Autodesk Inventor part; units mm, degrees
ref_plane "YZ Plane" through (0, 0, 0) normal (1, 0, 0) x (0, 1, 0)
ref_plane "XZ Plane" through (0, 0, 0) normal (0, 1, 0) x (-1, 0, 0)
ref_plane "XY Plane" through (0, 0, 0) normal (0, 0, 1) x (1, 0, 0)
sketch "Sketch1" plane through (0, 0, 0) normal (1, 0, 0) x (0, 1, 0)
  line L0 (0.3153, 51.2567) -> (-2.5847, 51.2567)
  line L1 (-2.5847, 51.2567) -> (-2.5847, -10.8433)
  line L2 (-2.5847, -10.8433) -> (0.3153, -10.8433)
  line L3 (0.3153, -10.8433) -> (0.3153, 51.2567)
  arc A0 (0.3153, 51.2567) -> (-0.0756, 57.3616) centre (-1.1163, 54.23) ccw
  arc A1 (-2.2756, 57.3196) -> (-2.5847, 51.2567) centre (-1.1371, 54.2222) ccw
  line L4 (-2.2756, 57.3196) -> (-2.2756, 56.2196)
  line L5 (-0.0756, 57.3616) -> (-0.0756, 56.2616)
  arc A2 (-2.2756, 56.2196) -> (-0.0756, 56.2616) centre (-1.1371, 54.2222) ccw
  arc A3 (-2.5847, -10.8433) -> (-2.5847, -16.9063) centre (-1.2354, -13.8748) ccw
  arc A4 (-0.3847, -16.0719) -> (-2.5847, -15.8063) centre (-1.2354, -13.8748) ccw
  arc A5 (-0.3847, -17.1719) -> (0.3153, -10.8433) centre (-1.2354, -13.8748) ccw
  line L6 (-2.5847, -15.8063) -> (-2.5847, -16.9063)
  line L7 (-0.3847, -16.0719) -> (-0.3847, -17.1719)
  point P0 (0, 0)
  dimension "d0" = 2.9
  dimension "d1" = 62.1
  dimension "d163" = 1.1
  dimension "d164" = 1.1
  dimension "d165" = 2.2
  dimension "d166" = 2.2991
  dimension "d167" = 3.3
  dimension "d168" = 3.3
  dimension "d171" = 6.063
  dimension "d172" = 6.1049
  dimension "d174" = 6.063
  dimension "d176" = 1.1
  dimension "d177" = 1.1
  dimension "d178" = 2.2
extrude "Extrusion1" add sketch "Sketch1" against normal blind 20
sketch "Sketch3" plane through (0, 0, 0) normal (1, 0, 0) x (0, 0, -1)
  line L0 (10.8433, -2.5847) -> (-51.2567, -2.5847)
  line L1 (-51.2567, 0.3153) -> (10.8433, 0.3153)
  line L2 (10.8433, 0.3153) -> (10.8433, -2.5847)
  line L3 (10.8433, -2.5847) -> (-51.2567, -2.5847)
  line L4 (-51.2567, -2.5847) -> (-51.2567, 0.3153)
  point P0 (0, 0)
extrude "Extrusion2" add sketch "Sketch3" along normal blind 42.1
sketch "Sketch4" plane through (42.1, 0, 0) normal (1, 0, 0) x (0, 0, -1)
  line L0 (10.8433, -2.5847) -> (-51.2567, -2.5847)
  line L1 (10.8433, -2.5847) -> (-51.2567, -2.5847)
  line L2 (-51.2567, -2.5847) -> (-51.2567, 0.3153)
  line L3 (-51.2567, 0.3153) -> (10.8433, 0.3153)
  line L4 (10.8433, 0.3153) -> (10.8433, -2.5847)
  arc A0 (-57.3196, -2.2756) -> (-51.2567, -2.5847) centre (-54.2222, -1.1371) ccw
  arc A1 (-57.3196, -2.2756) -> (-51.2567, -2.5847) centre (-54.2222, -1.1371) ccw
  arc A2 (-51.2567, 0.3153) -> (-57.3616, -0.0756) centre (-54.23, -1.1163) ccw
  arc A3 (-51.2567, 0.3153) -> (-57.3616, -0.0756) centre (-54.2286, -1.1372) ccw
  arc A4 (-56.2196, -2.2756) -> (-56.2616, -0.0756) centre (-54.2222, -1.1371) ccw
  arc A5 (-56.2196, -2.2756) -> (-56.2616, -0.0756) centre (-54.2286, -1.1372) ccw
  line L5 (-56.2196, -2.2756) -> (-57.3196, -2.2756)
  line L6 (-56.2196, -2.2756) -> (-57.3196, -2.2756)
  line L7 (-57.3616, -0.0756) -> (-56.2616, -0.0756)
  line L8 (-56.2616, -0.0756) -> (-57.3616, -0.0756)
  arc A6 (-57.3196, -2.2756) -> (-51.2567, -2.5847) centre (-54.2222, -1.1371) ccw
  line L9 (-51.2567, -2.5847) -> (-51.2567, 0.3153)
  arc A7 (-51.2567, 0.3153) -> (-57.3616, -0.0756) centre (-54.23, -1.1163) ccw
  arc A8 (-56.2196, -2.2756) -> (-56.2616, -0.0756) centre (-54.2222, -1.1371) ccw
  line L10 (-57.3196, -2.2756) -> (-56.2196, -2.2756)
  line L11 (-56.2616, -0.0756) -> (-57.3616, -0.0756)
  line L12 (-56.2616, -0.0756) -> (-57.3616, -0.0756)
  line L13 (-56.2616, -0.0756) -> (-57.3616, -0.0756)
  arc A9 (10.8433, -2.5847) -> (16.9063, -2.5847) centre (13.8748, -1.2354) ccw
  arc A10 (10.8433, -2.5847) -> (16.9063, -2.5847) centre (13.8748, -1.2354) ccw
  arc A11 (17.1719, -0.3847) -> (10.8433, 0.3153) centre (13.8748, -1.2354) ccw
  arc A12 (17.1719, -0.3847) -> (10.8433, 0.3153) centre (13.8748, -1.2354) ccw
  arc A13 (16.0719, -0.3847) -> (15.8063, -2.5847) centre (13.8748, -1.2354) ccw
  arc A14 (16.0719, -0.3847) -> (15.8063, -2.5847) centre (13.8748, -1.2354) ccw
  line L14 (15.8063, -2.5847) -> (16.9063, -2.5847)
  line L15 (16.0719, -0.3847) -> (17.1719, -0.3847)
extrude "Extrusion3" add sketch "Sketch4" along normal blind 20 contours L0 L2 L3 L4 | L4 A11 L15 A13 L14 A9 | A0 L5 A4 L7 A3 L2 | A3 A2
sketch "Sketch9" plane through (0, -2.5847, 51.2567) normal (0, 0, 1) x (1, 0, 0)
  line L0 (0, 2.9) -> (42.1, 2.9)
  line L1 (0, 2.9) -> (42.1, 2.9)
  line L2 (42.1, 2.9) -> (42.1, 0)
  line L3 (42.1, 0) -> (0, 0)
  line L4 (0, 0) -> (0, 2.9)
  point P0 (0, 2.5847)
extrude "Extrusion4" add sketch "Sketch9" along normal blind 0.001
sketch "Sketch10" plane through (-20, 0, 0) normal (-1, 0, 0) x (0, 0, 1)
  arc A0 (51.2567, -2.5847) -> (57.3196, -2.2756) centre (54.2222, -1.1371) ccw
  line L0 (-10.8433, 0.3153) -> (-10.8433, -2.5847)
  line L1 (51.2567, -2.5847) -> (-10.8433, -2.5847)
  line L2 (-10.8433, -2.5847) -> (-10.8433, 0.3153)
  line L3 (-10.8433, 0.3153) -> (51.2567, 0.3153)
  line L4 (51.2567, 0.3153) -> (51.2567, -2.5847)
  point P0 (0, 0)
  point P1 (-10.8433, -2.5847)
extrude "Extrusion5" add sketch "Sketch10" along normal blind 8.95
sketch "Sketch11" plane through (62.1, 0, 0) normal (1, 0, 0) x (0, 0, -1)
  line L0 (10.8433, -2.5847) -> (10.8433, 0.3153)
  arc A0 (-51.2567, 0.3153) -> (-57.3616, -0.0756) centre (-54.23, -1.1163) ccw
  line L1 (10.8433, -2.5847) -> (-51.2567, -2.5847)
  line L2 (-51.2567, -2.5847) -> (-51.2567, 0.3153)
  line L3 (-51.2567, 0.3153) -> (10.8433, 0.3153)
  line L4 (10.8433, 0.3153) -> (10.8433, -2.5847)
  point P0 (0, 0)
  point P1 (-57.2033, 0.3153)
  point P2 (10.8433, 0.3153)
extrude "Extrusion6" add sketch "Sketch11" along normal blind 8.95
sketch "Sketch12" plane through (0, -2.5847, 57.2567) normal (0, -1, 0) x (1, 0, 0)
  line L0 (-20, -6) -> (-30, -6)
  line L1 (-30, -68.1) -> (-30, -6)
  point P0 (-24.59, -14.57)
  dimension "d133" = 8.57
  dimension "d134" = 5.41
hole "Hole5" at (-24.59, -2.5847, 42.6867) direction (0, 1, 0) diameter 2.921 end through all
sketch "Sketch13" plane through (0, -2.5847, 57.2567) normal (0, -1, 0) x (1, 0, 0)
  line L0 (0, -6) -> (-20, -6)
  circle A0 centre (-24.59, -14.57) radius 1.4605
  point P0 (-11.33, -14.57)
  dimension "d135" = 8.57
  dimension "d136" = 13.26
hole "Hole6" at (-11.33, -2.5847, 42.6867) direction (0, 1, 0) diameter 2.921 end through all
sketch "Sketch14" plane through (0, -2.5847, 57.2567) normal (0, -1, 0) x (1, 0, 0)
  line L0 (-28.95, -68.1) -> (-28.95, -6)
  circle A0 centre (-24.59, -14.57) radius 1.4605
  point P0 (0, -57.2567)
  point P1 (-23.54, -59.5177)
  dimension "d137" = 5.41
  dimension "d138" = 44.96
hole "Hole7" at (-23.54, -2.5847, -2.2611) direction (0, 1, 0) diameter 2.921 end through all
sketch "Sketch15" plane through (0, -2.5847, 57.2567) normal (0, -1, 0) x (1, 0, 0)
  circle A0 centre (-11.33, -14.57) radius 1.4605
  circle A1 centre (-23.54, -59.5177) radius 1.4605
  point P0 (0, -57.2567)
  point P1 (-10.28, -59.53)
  dimension "d139" = 44.96
  dimension "d148" = 13.26
hole "Hole8" at (-10.28, -2.5847, -2.2733) direction (0, 1, 0) diameter 2.921 end through all
sketch "Sketch17" plane through (0, -2.5847, 57.2567) normal (0, -1, 0) x (1, 0, 0)
  line L0 (71.05, -6) -> (71.05, -68.1)
  line L1 (62.1, -6) -> (71.05, -6)
  point P0 (0, -57.2567)
  point P1 (65.64, -14.57)
  dimension "d142" = 5.41
  dimension "d147" = 8.57
hole "Hole10" at (65.64, -2.5847, 42.6867) direction (0, 1, 0) diameter 2.921 end through all
sketch "Sketch16" plane through (0, -2.5847, 57.2567) normal (0, -1, 0) x (1, 0, 0)
  circle A0 centre (65.64, -14.57) radius 1.4605
  line L0 (42.1, -6) -> (62.1, -6)
  point P0 (0, -57.2567)
  point P1 (52.38, -14.57)
  dimension "d144" = 13.26
  dimension "d146" = 8.57
hole "Hole9" at (52.38, -2.5847, 42.6867) direction (0, 1, 0) diameter 2.921 end through all
sketch "Sketch19" plane through (0, -2.5847, 57.2567) normal (0, -1, 0) x (1, 0, 0)
  circle A0 centre (65.64, -14.57) radius 1.4605
  line L0 (71.05, -6) -> (71.05, -68.1)
  point P0 (0, -57.2567)
  point P1 (65.64, -59.53)
  dimension "d141" = 44.96
  dimension "d143" = 5.41
hole "Hole12" at (65.64, -2.5847, -2.2733) direction (0, 1, 0) diameter 2.921 end through all
sketch "Sketch18" plane through (0, -2.5847, 57.2567) normal (0, -1, 0) x (1, 0, 0)
  circle A0 centre (52.38, -14.57) radius 1.4605
  circle A1 centre (65.64, -59.53) radius 1.4605
  point P0 (0, -57.2567)
  point P1 (52.38, -59.53)
  dimension "d140" = 44.96
  dimension "d145" = 13.26
hole "Hole11" at (52.38, -2.5847, -2.2733) direction (0, 1, 0) diameter 2.921 end through all
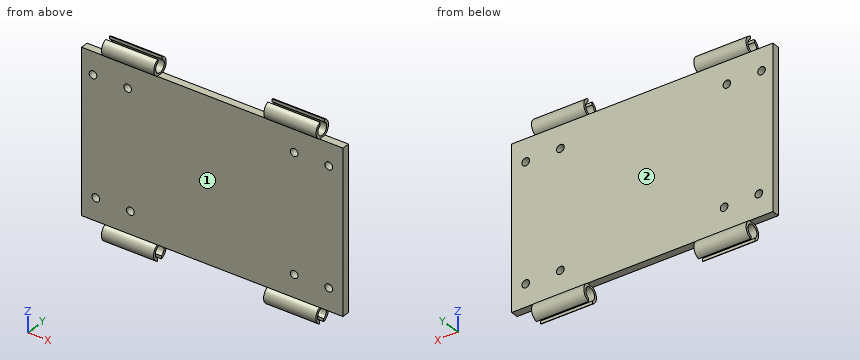
Design review of the part built by this model. Coordinates are the model's own, in mm. Face numbers are marked on the shaded views. A direction names the side the tool comes from. Coordinates: 2 decimals unless noted, no trailing zeros. Order: outer loops, then holes, each group sorted by start corner. A loop starts at its lowest first (then second) coordinate and runs counter-clockwise, first axis right, second up.
Item 1: For line 1 (Z direction, x = 65.64, y = -1.1); line 2 (Z direction, x = 52.38, y = -1.05); line 3 (Y direction, x = 28, z = 41), list the stretches that pass through material, from the lowest coordinate up.
Item 2: Take a section at D-D, the plane z = 24. Write out the cut boundary in (x, y), then the cut area to 3 significant figures.
Item 3: Take a section at A-A, the plane x = 52.38. Write out the cut boundary in (y, z), then the cut area to 3 significant figures.
Item 4: For pin 1 Ø5 at (x, z) = (32, 16.5) entering from +Y; pin 2 Ø2.5 at (x, y) = (-24.5, -1) entering from +Z; pin 3 Ø1.2 at (x, z) = (53, -16.5) entering from -Y, all flat-tipped, find the tip position at first contact; note any pin that passes through.
Item 5: For the marked faces 1 and 2, list the 3-axis set-ups (+Z, -Z, +X, -X, +Y, -Y) from which the entire face can be reached by the end or side of a thin tool; tool diameter is ignored.
Item 6: Take a section at B-B, the plane x = -15.5. Write out the cut boundary in (y, z), then the cut area to 3 significant figures.
Item 7: Take a section at C-C, the plane x = 65.64. Write out the cut boundary in (y, z), then the cut area to 3 significant figures.
The answers:
1. line 1: z = -10.84 to -3.73, -0.81 to 41.23, 44.15 to 51.26
1. line 2: z = -11.53 to -3.73, -0.81 to 41.23, 44.15 to 51.92
1. line 3: y = -2.58 to 0.32
2. outline: (-28.95, -2.58) - (71.05, -2.58) - (71.05, 0.32) - (-28.95, 0.32) - close
2. area: 290 mm2
3. outline: (-2.58, -16.91) - (-2.58, -15.81) arc R2.36 cw (long way) to (-0.38, -16.07) - (-0.38, -17.17) arc R3.41 ccw to (0.32, -10.84) - (0.32, -3.73) - (-2.58, -3.73) - (-2.58, -10.84) arc R3.32 ccw to start; (-2.58, -0.81) - (0.32, -0.81) - (0.32, 41.23) - (-2.58, 41.23) - close; (-2.58, 44.15) - (0.32, 44.15) - (0.32, 51.26) arc R3.3 ccw to (-0.08, 57.36) - (-0.08, 56.26) arc R2.3 cw (long way) to (-2.28, 56.22) - (-2.28, 57.32) arc R3.3 ccw to (-2.58, 51.26) - close
3. area: 193 mm2
4. pin 1: stops at y = 0.32
4. pin 2: stops at z = 51.26
4. pin 3: stops at y = -3.86
5. face 1: +X, -X, -Y
5. face 2: +X, -X, +Y
6. outline: (-2.58, -16.91) - (-2.58, -15.81) arc R2.36 cw (long way) to (-0.38, -16.07) - (-0.38, -17.17) arc R3.41 ccw to (0.32, -10.84) - (0.32, 51.26) arc R3.3 ccw to (-0.08, 57.36) - (-0.08, 56.26) arc R2.3 cw (long way) to (-2.28, 56.22) - (-2.28, 57.32) arc R3.3 ccw to (-2.58, 51.26) - (-2.58, -10.84) arc R3.32 ccw to start
6. area: 210 mm2
7. outline: (-2.58, -10.84) - (0.32, -10.84) - (0.32, -3.73) - (-2.58, -3.73) - close; (-2.58, -0.81) - (0.32, -0.81) - (0.32, 41.23) - (-2.58, 41.23) - close; (-2.58, 44.15) - (0.32, 44.15) - (0.32, 51.26) - (-2.58, 51.26) - close
7. area: 163 mm2
